Autodesk Inventor part; units mm, degrees
ref_plane "YZ Plane" through (0, 0, 0) normal (1, 0, 0) x (0, 1, 0)
ref_plane "XZ Plane" through (0, 0, 0) normal (0, 1, 0) x (-1, 0, 0)
ref_plane "XY Plane" through (0, 0, 0) normal (0, 0, 1) x (1, 0, 0)
ref_plane "Work Plane1" through (-6.4883, -6.1632, -131.5017) normal (0, 1, 0) x (-1, 0, 0)
sketch "Sketch1" plane through (-6.4883, -6.1632, -131.5017) normal (0, 1, 0) x (-1, 0, 0)
  line L0 (-2, -18) -> (-2, 0)
  line L1 (-2, 0) -> (-7.4816, 0)
  line L2 (-22.4693, -8.5807) -> (-7.4816, 0)
  line L3 (-6.2906, -18) -> (-22.4693, -8.5807)
  line L4 (-2, -18) -> (-6.2906, -18)
  point P0 (-6.4883, 131.5017)
extrude "Extrusion1" add sketch "Sketch1" along normal blind 8
sketch "Sketch2" plane through (0, 0, 0) normal (1, 0, 0) x (0, 1, 0)
  line L0 (-6.1632, -140.0824) -> (1.8368, -140.0824)
  circle A0 centre (-2.1632, -140.0824) radius 3
  point P0 (0, 0)
  dimension "d2" = 6
extrude "Extrusion2" cut sketch "Sketch2" along normal through all both and the other way through all
sketch "Sketch3" plane through (-6.4883, 1.8368, -131.5017) normal (0, 1, 0) x (1, 0, 0)
  line L0 (2, 18) -> (2, 0)
  line L1 (17.3164, 11.5807) -> (22.4693, 8.5807)
  line L2 (2, 0) -> (22.4693, 0)
  line L3 (22.4693, 0) -> (22.4693, 8.5807)
  line L4 (22.4693, 8.5807) -> (2, 8.5807)
  line L5 (2, 8.5807) -> (2, 0)
  point P0 (6.4883, -131.5017)
extrude "Extrusion3" cut sketch "Sketch3" against normal through all
properties part number "Wire_Clossing"
Build history of the part. All positions in model axes, mm. Give positions to 0.01 mm unless a question says otherwise; leave off trailing zeros. Order: outer loops, then holes, each group sorted by start corner. A loop starts at its lowest first (then second) coordinate and runs counter-clockwise, first axis right, second up. Notation, with made-up numbers: M -14.5,-40 L 36.5,-40 A12 ccw 36.5,-24 Z; hole C -13,19 d2. An arc over 180 degrees is marked long. Put each result on its own line as item: value.
Item 1: Slice it at A-A, the plane x = -3. Write the cut outline in (y, z), plus the area to 3 significant figures.
From the geometry:
outline: M -6.16,-149.5 L 1.84,-149.5 L 1.84,-140.08 L 0.84,-140.08 A3 cw -5.16,-140.08 L -6.16,-140.08 Z
area: 61.2 mm2
Item 2: Slice it at D-D, the plane x = 9. Write the cut outline in (y, z), plus the area to 3 significant figures.
From the geometry:
outline: M -6.16,-144.15 L 1.84,-144.15 L 1.84,-140.08 L 0.84,-140.08 A3 cw -5.16,-140.08 L -6.16,-140.08 Z
area: 18.4 mm2
Item 3: Flat gauge pins, fed straight in: pin 1 Ø1.5 at (x, y) = (10, -3) entering from -Z; pin 2 Ø3 at (y, z) = (0.5, -144) entering from +X; pin 3 Ø2 at (x, y) = (1.5, -2) entering from -Z. Where does each tip first touch, or does it go through?
From the geometry:
pin 1: stops at z = -144
pin 2: stops at x = 11.83
pin 3: stops at z = -149.1
Item 4: Probe line 1 (Y direction, x = 8, z = -140.5); line 2 (Y direction, x = 6.25, z = -141.5); line 3 (X direction, y = -0.5, z = -144.75). List the from-to ranges inside material, lowest first. Write a range as [from, to].
From the geometry:
line 1: y = [-6.16, -5.13], [0.81, 1.84]
line 2: y = [-6.16, -4.81], [0.48, 1.84]
line 3: x = [-4.49, 7.96]
Item 5: Slice it at C-C, the plane z = -146.5. Write the cut outline in (x, y), plus the area to 3 significant figures.
From the geometry:
outline: M -4.49,-6.16 L 4.96,-6.16 L 4.96,1.84 L -4.49,1.84 Z
area: 75.6 mm2
Item 6: Slice it at B-B, the plane y = -5.5. Write the cut outline in (x, z).
From the geometry:
outline: M -4.49,-149.5 L -0.2,-149.5 L 15.98,-140.08 L -4.49,-140.08 Z
